Work out the finished part from the listing and answer in its coordinate system (mm). Round coordinates to 2 decimals unless told otherwise and drop trailing zeros. Order: outer loops, then holes, each group sorted by start corner. A loop starts at its lowest first (then second) coordinate and runs counter-clockwise, first axis right, second up. Notation, with made-up numbers: (66.25, -29) - (80.25, -29) arc R16 ccw to (80.25, -18) - close; hole circle Ø2 at (42, 29.5). An arc over 180 degrees is marked (long way). Answer in a Markdown table with one row per item.
from build123d import *

# Parameters (mm, degrees)
SKETCH1_W           = 56
SKETCH1_H           = 666.6
DOME1_FACE_RADIUS   = 56
DOME1_HEIGHT        = 166.665
SKETCH3_W           = 15
SKETCH3_H           = 100
BOSS_EXTRUDE1_DEPTH = 66


with BuildPart() as part:
    # Sketch1 → Revolve1 (revolve)
    with BuildSketch(Plane.XY, mode=Mode.PRIVATE) as revolve1_sk:
        with Locations((28, -333.3)):
            Rectangle(SKETCH1_W, SKETCH1_H)
    revolve(revolve1_sk.sketch.rotate(Axis((0, 0, 0), (0, -1, 0)), 180), axis=Axis((0, 0, 0), (0, -1, 0)))

    # Dome1: an elliptical dome of height H over a round flat face of radius A is half a spheroid: the quarter ellipse of half axes A and H revolved about the face's axis
    with BuildSketch(Plane((0, 0, 0), x_dir=(0, 0, -1), z_dir=(1, 0, 0)), mode=Mode.PRIVATE) as dome1_quarter:
        Ellipse(DOME1_FACE_RADIUS, DOME1_HEIGHT)
        Rectangle(DOME1_FACE_RADIUS, DOME1_HEIGHT, align=(Align.MIN, Align.MIN), mode=Mode.INTERSECT)
    revolve(dome1_quarter.sketch, axis=Axis((0, 0, 0), (0, 1, 0)))

    # Sketch2 → Revolve2 (revolve)
    with BuildSketch(Plane.XY, mode=Mode.PRIVATE) as revolve2_sk:
        with BuildLine():
            Line((19.405267456, -666.6), (19.019237886, -667.268622827))
            ThreePointArc((19.019237886, -667.268622827), (16.022225211, -674.504051474), (15, -682.268622827))
            Line((15, -682.268622827), (15, -682.579307175))
            ThreePointArc((15, -682.579307175), (15.711119786, -689.072495593), (17.810766389, -695.257855027))
            Line((17.810766389, -695.257855027), (66, -798.6))
            Line((66, -798.6), (0, -798.6))
            Line((0, -798.6), (0, -666.6))
            Line((0, -666.6), (19.405267456, -666.6))
        make_face()
    revolve(revolve2_sk.sketch.rotate(Axis((0, -1354.267338739, 0), (0, 1, 0)), 90), axis=Axis((0, -1354.267338739, 0), (0, 1, 0)))

    # Sketch3 → Boss-Extrude1 (add)
    with BuildSketch(Plane.XY):
        with Locations((0, -366.6)):
            Rectangle(SKETCH3_W, SKETCH3_H)
    extrude(amount=BOSS_EXTRUDE1_DEPTH)


solid = part.part
1) The mould has two halves that part along Y. Classify faces 1 (the face through (-1, -798.6, 1)), 2 (the face through (0, -366, 66)), 3 (the face through (-12.648, -682.426, -8.064)): released by +Y, released by -Y, zero draft, split by the parting line, or undercut.
Filled in:
| item | result |
|---|---|
| face 1 | released by -Y |
| face 2 | zero draft |
| face 3 | undercut |
2) Find section A-A, the plane y = -303.5. Give the vertices of the cut face in (x, z), then the cut area to 3 significant figures.
Filled in:
| item | result |
|---|---|
| outline | circle Ø112 at (0, 0) |
| area | 9,850 mm^2 |
3) Find the intervals of material crossed by probe 1 along Z at (x, y) = (-3.5, -589); probe 2 along Y at (x, z) = (-25, 15.5); probe 3 along Y at (x, z) = (20.5, -19.5), in increasing order. Write a range as from..to.
Filled in:
| item | result |
|---|---|
| probe 1 | z = -55.89..55.89 |
| probe 2 | y = -798.6..-720.14, -666.6..141.82 |
| probe 3 | y = -798.6..-717.74, -666.6..143.83 |
4) Each of these flat-tipped pins is pushed along its axis until it touches: pin 1 (5 mm diameter, centred on x = -16.5, y = -553, fed in from +Z); pin 2 (12 mm diameter, centred on x = -4, y = -178.5, fed in from +Z); pin 3 (4 mm diameter, centred on y = -593.5, z = -39, fed in from +X). Where does it stop, or does it pass through?
Filled in:
| item | result |
|---|---|
| pin 1 | stops at z = 54.22 |
| pin 2 | stops at z = 56 |
| pin 3 | stops at x = 42.04 |
